```python
from build123d import *

# Parameters (mm, degrees)
SKETCH1_R           = 11.1125
BOSS_EXTRUDE1_DEPTH = 4.7625
SKETCH2_R           = 6.35
CUT_EXTRUDE1_DEPTH  = 17.421227687


with BuildPart() as part:
    # Sketch1 → Boss-Extrude1 (new body)
    with BuildSketch(Plane.XY):
        with Locations(Location((0, 0, 0), (0, 0, 180))):
            Circle(SKETCH1_R)
    extrude(amount=BOSS_EXTRUDE1_DEPTH)

    # Sketch2 → Cut-Extrude1 (cut, through all)
    with BuildSketch(Plane.XY.offset(4.7625)):
        Circle(SKETCH2_R)
    extrude(amount=-CUT_EXTRUDE1_DEPTH, mode=Mode.SUBTRACT)

    # Sketch3 → Cut-Revolve1 (revolve, cut)
    with BuildSketch(Plane.XY.offset(2.38125), mode=Mode.PRIVATE) as cut_revolve1_sk:
        Polygon((1.193659919, -11.1125), (1.171897939, 11.1125), (0, 11.1125), (0, -11.1125), align=None)
    revolve(cut_revolve1_sk.sketch.rotate(Axis((0, 11.1125, 2.38125), (0, -1, 0)), 224.092612296), axis=Axis((0, 11.1125, 2.38125), (0, -1, 0)), mode=Mode.SUBTRACT)


solid = part.part
```
Verification items for the finished model (mm, model axes). Round coordinates to 2 decimals unless told otherwise and drop trailing zeros. Write each loop counter-clockwise with the first axis right and the second up, starting at its lowest first coordinate (ties: lowest second). Pieces come first, ordered by that corner, then holes. Notation, with made-up numbers: (37, -12) -> (78, -12) arc R30 cw to (78, 20) -> close; hole circle Ø7 at (-2.75, -16.5). An arc over 180 degrees is marked (long way). Write each question's results on one line, items separated by ' | '. Start each with the question number.
1. Cross-section at D-D (y = -7). Enter the section's corners in (x, z), then the cut area to 3 significant figures.
2. Cross-section at B-B (x = 5). Enter the section's corners in (y, z), then the cut area to 3 significant figures.
3. Draft check along X on faces 1 (the flat face through (-5, 5, 0)), 2 (the cylindrical face through (-1.38, -6.2, 2.41)), 3 (the cylindrical face through (8.2, -7.5, 2.3)). Enter one of: +X half, -X half, draft (parallel to the pull), parting line (faces both ways), or undercut.
4. Material ranges on probe 1 along Y at (x, z) = (-3.5, 0.2); probe 2 along Y at (x, z) = (0, 3.85), recorded low to high. Write a range as from..to.
5. Cross-section at A-A (y = 0). Enter the section's corners in (x, z), then the cut area to 3 significant figures.
6. Depth check by flat-ended pin: P1, Ø1, axis at x = -8.5, z = 2.5, coming from the -Y side; P2, Ø1.5, axis at x = -9, z = 3, coming from the +Y side. Enter the tip coordinate at first touch or a pass-through.
Solutions:
1) outline: (-8.63, 0) -> (8.63, 0) -> (8.63, 4.76) -> (-8.63, 4.76) -> close; hole circle Ø2.38 at (0, 2.38) | area: 77.8 mm2
2) outline: (-9.92, 0) -> (-3.91, 0) -> (-3.91, 4.76) -> (-9.92, 4.76) -> close; (3.91, 0) -> (9.92, 0) -> (9.92, 4.76) -> (3.91, 4.76) -> close | area: 57.2 mm2
3) face 1: draft | face 2: undercut | face 3: parting line
4) probe 1: y = -10.55..-5.3, 5.3..10.55 | probe 2: y = -11.11..-6.35, 6.35..11.11
5) outline: (-11.11, 0) -> (-6.35, 0) -> (-6.35, 4.76) -> (-11.11, 4.76) -> close; (6.35, 0) -> (11.11, 0) -> (11.11, 4.76) -> (6.35, 4.76) -> close | area: 45.4 mm2
6) P1: stops at y = -7.71 | P2: stops at y = 7.44
